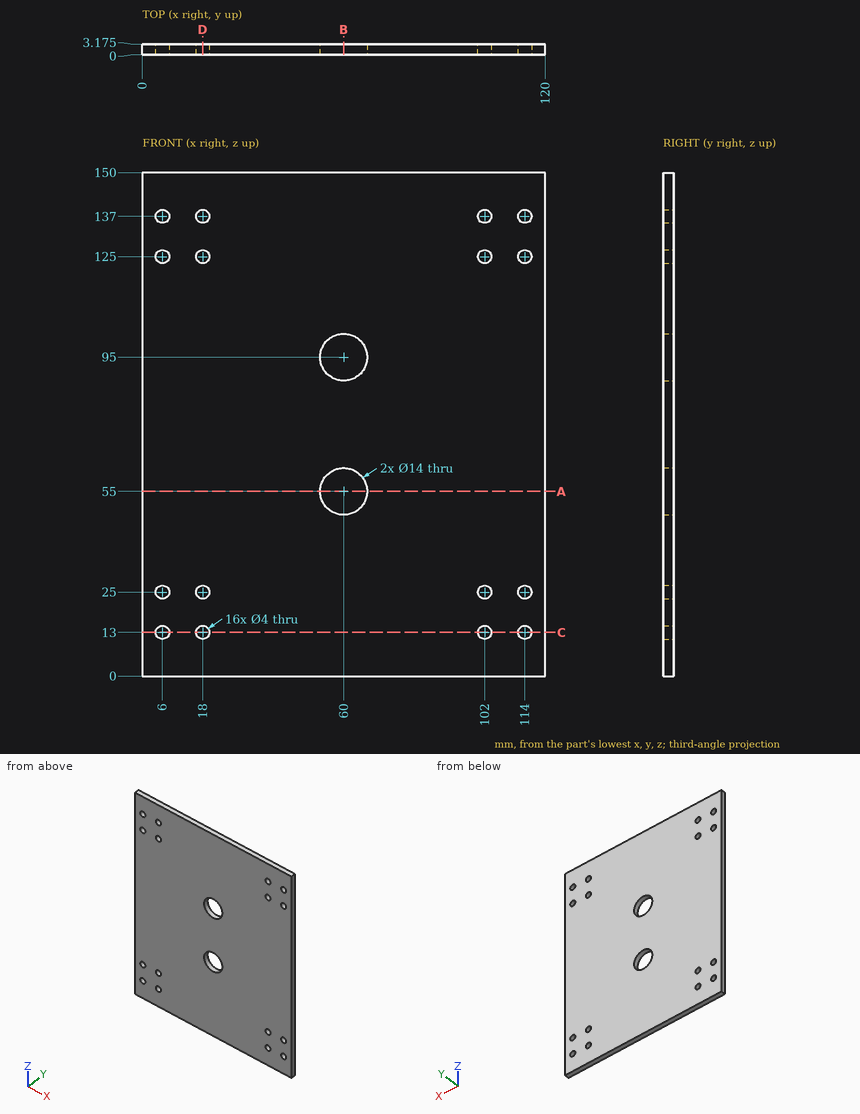
Job drawing, mm, ordinate dimensions from the low corner. One solid piece. Round coordinates to 2 decimals unless told otherwise and drop trailing zeros. Write each loop counter-clockwise with the first axis right and the second up, starting at its lowest first coordinate (ties: lowest second). Pieces come first, ordered by that corner, then holes.
1) Drill centre lines: probe 1 along Z at (x, y) = (60, 1.1); probe 2 along Z at (x, y) = (6, 1.5); probe 3 along X at (y, z) = (1.9, 137). Where is each one in solid material? Low to high.
2) Pin check, flat tip, straight feed: pin 1 (11 mm diameter, centred on x = 60, z = 95, fed in from -Y). Stop position of the tip, or through.
3) Band-saw the part on C-C, the plane z = 13. List the corners of the cut face in (x, y) (3 decimals).
4) Band-saw the part on D-D, the plane x = 18. List the corners of the cut face in (y, z) (3 decimals), and give its area (3 significant figures).
5) Band-saw the part on A-A, the plane z = 55. List the corners of the cut face in (x, y) (3 decimals).
6) Band-saw the part on B-B, the plane x = 60. List the corners of the cut face in (y, z) (3 decimals), and give its area (3 significant figures).
Ans:
1. probe 1: z = 0 to 48, 62 to 88, 102 to 150
1. probe 2: z = 0 to 11, 15 to 23, 27 to 123, 127 to 135, 139 to 150
1. probe 3: x = 0 to 4, 8 to 16, 20 to 100, 104 to 112, 116 to 120
2. pin 1: passes through
3. outline: (0, 0) - (4, 0) - (4, 3.175) - (0, 3.175) - close; (8, 0) - (16, 0) - (16, 3.175) - (8, 3.175) - close; (20, 0) - (100, 0) - (100, 3.175) - (20, 3.175) - close; (104, 0) - (112, 0) - (112, 3.175) - (104, 3.175) - close; (116, 0) - (120, 0) - (120, 3.175) - (116, 3.175) - close
4. outline: (0, 0) - (3.175, 0) - (3.175, 11) - (0, 11) - close; (0, 15) - (3.175, 15) - (3.175, 23) - (0, 23) - close; (0, 27) - (3.175, 27) - (3.175, 123) - (0, 123) - close; (0, 127) - (3.175, 127) - (3.175, 135) - (0, 135) - close; (0, 139) - (3.175, 139) - (3.175, 150) - (0, 150) - close
4. area: 425 mm2
5. outline: (0, 0) - (53, 0) - (53, 3.175) - (0, 3.175) - close; (67, 0) - (120, 0) - (120, 3.175) - (67, 3.175) - close
6. outline: (0, 0) - (3.175, 0) - (3.175, 48) - (0, 48) - close; (0, 62) - (3.175, 62) - (3.175, 88) - (0, 88) - close; (0, 102) - (3.175, 102) - (3.175, 150) - (0, 150) - close
6. area: 387 mm2
